The listing builds one solid part. Answer for the finished solid, in the listing's coordinates (mm). Coordinates: 2 decimals unless noted, no trailing zeros. Order: outer loops, then holes, each group sorted by start corner. A loop starts at its lowest first (then second) coordinate and runs counter-clockwise, first axis right, second up. Notation, with made-up numbers: (87.5, -23.75) -> (113.5, -23.75) arc R23 cw to (113.5, -14.75) -> close; hole circle Ø1 at (29, 18). An arc over 180 degrees is marked (long way). Put each result on its own line as item: value. Start each with the question number.
```python
from build123d import *

# Parameters (mm, degrees)
BOSS_EXTRUDE1_DEPTH = 2.6
CAVITY1_OUTLINE_R   = 1.05
CAVITY1_DEPTH       = 2.6


# Read off the part's stored shape, not the designer's step: Cavity1
with BuildPart() as part:
    # Sketch1 → Boss-Extrude1 (new body)
    with BuildSketch(Plane.XY):
        Polygon((20.678672923, 94.689954591), (-2.25890757, 73.836480034), (-2.25890757, 21.810264808), (19.661402647, -0.110045409), (69.603511937, -0.110045409), (92.54109243, 20.743429149), (92.54109243, 72.769644374), (70.620782213, 94.689954591), align=None)
    extrude(amount=BOSS_EXTRUDE1_DEPTH)

    # Cavity1 outline → Cavity1 (cut)
    with BuildSketch(Plane.XY):
        with Locations((34.534490712, 57.896556309)):
            Circle(CAVITY1_OUTLINE_R)
        with Locations((34.534490712, 36.683352873)):
            Circle(CAVITY1_OUTLINE_R)
        with Locations((55.747694148, 57.896556309)):
            Circle(CAVITY1_OUTLINE_R)
        with Locations((55.747694148, 36.683352873)):
            Circle(CAVITY1_OUTLINE_R)
    extrude(amount=CAVITY1_DEPTH, mode=Mode.SUBTRACT)


solid = part.part
```
(1) The part is cut by section A-A on z = 0.4. Determine the outline of the cut face in (x, y), plus the area to 3 significant figures.
(2) The part is cut by section C-C on x = 83. Determine the outline of the cut face in (y, z), plus the area to 3 significant figures.
(3) Find the intervals of material crossed by L1, parallel to X at y = 82, z = 2; L2, parallel to Y at x = 4, z = 1.4; L3, parallel to X at y = 76, z = 1.2, in increasing order.
(4) For a pull along Y with two mould halves and no side action, classify faces 1 (the flat face through (46, 94.69, 1)), 2 (the flat face through (44, 48, 0)), 3 (the cylindrical face through (56.75, 58.21, 1.28)), 4 (the flat face through (44, -0.11, 1)) as released by +Y, released by -Y, zero draft, split by the parting line, or undercut.
(5) The part is cut by section B-B on y = 13. Determine the outline of the cut face in (x, z).
Worked out:
1. outline: (-2.26, 21.81) -> (19.66, -0.11) -> (69.6, -0.11) -> (92.54, 20.74) -> (92.54, 72.77) -> (70.62, 94.69) -> (20.68, 94.69) -> (-2.26, 73.84) -> close; hole circle Ø2.1 at (34.53, 36.68); hole circle Ø2.1 at (34.53, 57.9); hole circle Ø2.1 at (55.75, 36.68); hole circle Ø2.1 at (55.75, 57.9)
1. area: 8,010 mm2
2. outline: (12.07, 0) -> (82.31, 0) -> (82.31, 2.6) -> (12.07, 2.6) -> close
2. area: 183 mm2
3. L1: 6.72 to 83.31
3. L2: 15.55 to 79.53
3. L3: 0.12 to 89.31
4. face 1: released by +Y
4. face 2: zero draft
4. face 3: undercut
4. face 4: released by -Y
5. outline: (6.55, 0) -> (84.02, 0) -> (84.02, 2.6) -> (6.55, 2.6) -> close
